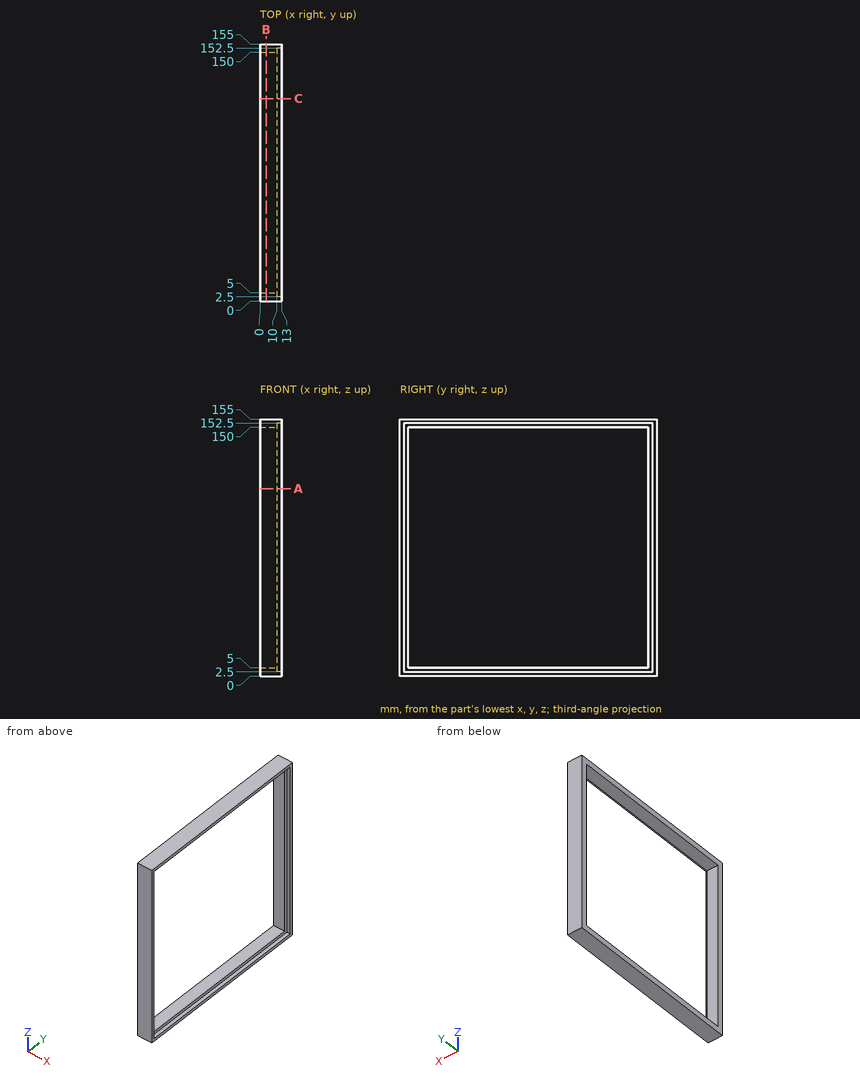
Job drawing, mm, ordinate dimensions from the low corner. One solid piece. Coordinates: 2 decimals unless noted, no trailing zeros. Order: outer loops, then holes, each group sorted by start corner. A loop starts at its lowest first (then second) coordinate and runs counter-clockwise, first axis right, second up. Notation, with made-up numbers: M -20,22.25 L 16,22.25 A15 ccw 16,27.25 Z; hole C 3.25,0 d7. An arc over 180 degrees is marked long. Answer as CSV lines item,"result".
(1) Band-saw the part on B-B, the plane x = 3.5. List the corners of the cut face in (y, z).
Geometry says:
outline,"M 0,0 L 155,0 L 155,155 L 0,155 Z; hole M 5,5 L 150,5 L 150,150 L 5,150 Z"
(2) Band-saw the part on A-A, the plane z = 113. List the corners of the cut face in (x, y).
Geometry says:
outline,"M 0,0 L 13,0 L 13,2.5 L 10,2.5 L 10,5 L 0,5 Z; M 0,150 L 10,150 L 10,152.5 L 13,152.5 L 13,155 L 0,155 Z"
(3) Wall check: line 1 along Y through (x, z) = (9.5, 26.5); line 2 along Z through (x, y) = (10.25, 27). Give the ranges that are in metal, low to high.
Geometry says:
line 1,"y = 0 to 5, 150 to 155"
line 2,"z = 0 to 2.5, 152.5 to 155"
